from build123d import *

# Parameters (mm, degrees)
SKETCH_1_W          = 35
SKETCH_1_H          = 20
EXTRUDE_1_DEPTH     = 20
CUT_EXTRUDE_1_DEPTH = 20
CUT_EXTRUDE_2_DEPTH = 32
CUT_EXTRUDE_3_DEPTH = 10
CUT_EXTRUDE_4_DEPTH = 19


with BuildPart() as part:
    # 草圖1 → 填料-伸長1 (new body)
    with BuildSketch(Plane(origin=(0, 0, 0), x_dir=(1, 0, 0), z_dir=(0, 1, 0))):
        Rectangle(SKETCH_1_W, SKETCH_1_H)
    extrude(amount=EXTRUDE_1_DEPTH)

    # 草圖2 → 除料-伸長1 (cut)
    with BuildSketch(Plane.XY.offset(10)):
        Polygon((17.5, 20), (-2.5, 20), (17.5, 10), align=None)
    extrude(amount=-CUT_EXTRUDE_1_DEPTH, mode=Mode.SUBTRACT)

    # 草圖3 → 除料-伸長2 (cut)
    with BuildSketch(Plane(origin=(0, 0, 0), x_dir=(1, 0, 0), z_dir=(0, 1, 0))):
        Polygon((-2.5, -10), (17.5, -10), (17.5, 0), align=None)
    extrude(amount=CUT_EXTRUDE_2_DEPTH, mode=Mode.SUBTRACT)

    # 草圖4 → 除料-伸長3 (cut)
    with BuildSketch(Plane(origin=(0, 20, 0), x_dir=(1, 0, 0), z_dir=(0, 1, 0))):
        Polygon((17.5, 0), (-2.5, 0), (-2.5, -10), align=None)
    extrude(amount=-CUT_EXTRUDE_3_DEPTH, mode=Mode.SUBTRACT)

    # 草圖5 → 除料-伸長4 (cut)
    with BuildSketch(Plane(origin=(-2.5, 0, 0), x_dir=(0, 0, -1), z_dir=(1, 0, 0))):
        Polygon((0, 20), (-10, 20), (-10, 10), align=None)
    extrude(amount=-CUT_EXTRUDE_4_DEPTH, mode=Mode.SUBTRACT)


solid = part.part
The listing builds one solid part. Answer for the finished solid, in the listing's coordinates (mm). A direction names the side the tool comes from. Coordinates: 2 decimals unless noted, no trailing zeros. Loops run counter-clockwise (first coordinate to the right, second up) from the corner with the lowest first, then second, coordinate; pieces in that order, holes last.
1) A tool of negligible diameter and unlimited length cuts with its end or side. For faces 1 (the face through (7.36, 15.07, -4.93)), 2 (the face through (5, 10, 4)), from which of +Z, -Z, +X, -X, +Y, -Y can it reach the whole face along a straight path? Write none if from no direction.
2) Find section D-D on x = -5. Write down the section's boundary in (y, z).
3) Flat-ended cylindrical pins translate along their axes: pin 1 Ø11 at (y, z) = (13, 5.5) entering from +X; pin 2 Ø5 at (x, z) = (-6, 3.5) entering from +Y; pin 3 Ø1 at (x, z) = (-6, 8) entering from +Y. Find the tip coordinate at first contact, or state that the pin passes through.
4) Find section A-A on x = 8.5. Write down the section's boundary in (y, z), then the cut area to 3 significant figures.
5) Find section C-C on z = -5.75. Write down the section's boundary in (x, y), then the cut area to 3 significant figures.
6) Find section B-B on y = 18.75. Write down the section's boundary in (x, z), then the cut area to 3 significant figures.
7) Find the intervals of material crossed by L1, parallel to Y at x = 1, z = 0.5; L2, parallel to X at y = 10.5, z = 4; L3, parallel to Y at x = 11.5, z = -6.5, in increasing order.
Values:
1. face 1: +Z, -Z, +X, +Y
1. face 2: +Z, +X, +Y
2. outline: (0, -10) - (20, -10) - (20, 0) - (10, 10) - (0, 10) - close
3. pin 1: stops at x = 15.72
3. pin 2: stops at y = 19
3. pin 3: stops at y = 12.5
4. outline: (0, -10) - (14.5, -10) - (14.5, 0) - (10, 0) - (10, 4.5) - (0, 4.5) - close
4. area: 190 mm2
5. outline: (-17.5, 0) - (17.5, 0) - (17.5, 10) - (-2.5, 20) - (-17.5, 20) - close
5. area: 600 mm2
6. outline: (-17.5, -10) - (0, -10) - (0, 0) - (-2.5, 0) - (-2.5, 1.25) - (-17.5, 1.25) - close
6. area: 194 mm2
7. L1: y = 0 to 10
7. L2: x = -17.5 to -2.5
7. L3: y = 0 to 13
